Check sheet for the modelled part. Datum: model origin and axes. Units: mm. A direction names the side the tool comes from. Give positions to 0.01 mm unless a question says otherwise; leave off trailing zeros. Order: outer loops, then holes, each group sorted by start corner. A loop starts at its lowest first (then second) coordinate and runs counter-clockwise, first axis right, second up.
```python
from build123d import *

# Parameters (mm, degrees)
F1_DEPTH  = 16
F2_W      = 70
F2_H      = 3
F3_DEPTH  = 2
F4_W      = 50
F4_H      = 14
F5_DEPTH  = 2
F6_R      = 1
F9_DEPTH  = 2
F11_DEPTH = 25
F13_D     = 4
F13_DEPTH = 50
F13_TIP   = 1.2017212381
F14_R     = 3
F14_R_2   = 2
F15_DEPTH = 5
F16_R     = 3


# Not quite as in the source:
# - a pattern or mirror of a feature is missing from the dataset's text; its kind, count and spacing are read off the source's solid


with BuildPart() as f1:
    # F0 (on Front) → F1 (new body)
    with BuildSketch(Plane.XZ):
        with BuildLine():
            Line((94, 11), (0, 11))
            ThreePointArc((0, 11), (-11, 0), (0, -11))
            Line((0, -11), (19, -11))
            ThreePointArc((19, -11), (21.7681124643, -11.8361612201), (23.6103896104, -14.064978646))
            ThreePointArc((23.6103896104, -14.064978646), (47.8977113224, -44.6078392712), (84.5520957277, -57.9942665386))
            ThreePointArc((84.5520957277, -57.9942665386), (89.6419160729, -59.3768457194), (93.8590048523, -62.5444881493))
            Line((93.8590048523, -62.5444881493), (95.1549842887, -61))
            ThreePointArc((95.1549842887, -61), (90.3976747979, -57.5207528796), (84.7034264019, -56))
            ThreePointArc((84.7034264019, -56), (49.0672193413, -42.9854179344), (25.4545454545, -13.2909701044))
            ThreePointArc((25.4545454545, -13.2909701044), (22.87535745, -10.1706257081), (19, -9))
            Line((19, -9), (0, -9))
            ThreePointArc((0, -9), (-9, 0), (0, 9))
            Line((0, 9), (94, 9))
            Line((94, 9), (94, 11))
        make_face()
    extrude(amount=F1_DEPTH)

    # F2 (on face) → F3 (join)
    with BuildSketch(Plane.XY.offset(11)):
        with Locations((59, -17.5)):
            Rectangle(F2_W, F2_H)
    extrude(amount=-F3_DEPTH)

    # F4 (on face) → F5 (join)
    with BuildSketch(Plane.XZ.offset(19)):
        with Locations((69, 4)):
            Rectangle(F4_W, F4_H)
    extrude(amount=-F5_DEPTH)

    # F6
    f6_edges = [f1.edges().sort_by_distance(p)[0] for p in [
        (59, -19, 11),
        (69, -17, 9),
    ]]
    fillet(f6_edges, radius=F6_R)

    # F7: F1 across plane


with BuildPart() as f1_1:
    add(f1.part)
    add(f1.part.mirror(Plane.XZ))

    # F8 (on face) → F9 (cut)
    with BuildSketch(Plane.XY.offset(11)):
        with BuildLine():
            Line((94, 12), (34, 12))
            ThreePointArc((34, 12), (22, 0), (34, -12))
            Line((34, -12), (94, -12))
            Line((94, -12), (94, 12))
        make_face()
    extrude(amount=-F9_DEPTH, mode=Mode.SUBTRACT)

    # F10 (on face) → F11 (cut)
    with BuildSketch(Plane.XZ.offset(19)):
        with BuildLine():
            ThreePointArc((50, 5), (47, 2), (50, -1))
            Line((50, -1), (70, -1))
            ThreePointArc((70, -1), (73, 2), (70, 5))
            Line((70, 5), (50, 5))
        make_face()
    extrude(amount=-F11_DEPTH, mode=Mode.SUBTRACT)

    # F13
    with Locations(Plane.XZ.offset(19)):
        with Locations((80, 3)):
            Hole(F13_D / 2, depth=F13_DEPTH)
            with Locations((0, 0, -(F13_DEPTH + F13_TIP / 2))):  # 118° drill point
                Cone(0, F13_D / 2, F13_TIP, mode=Mode.SUBTRACT)

    # F14 (on face) → F15 (join)
    with BuildSketch(Plane(origin=(0, -17, 0), x_dir=(-1, 0, 0), z_dir=(0, 1, 0))):
        with Locations((-80, 3)):
            Circle(F14_R)
        with Locations((-80, 3)):
            Circle(F14_R_2, mode=Mode.SUBTRACT)
    f15 = extrude(amount=F15_DEPTH)

    # F15_copies: F15 across plane
    add(f15.mirror(Plane.ZX))

    # F16
    f16_edges = [f1_1.edges().sort_by_distance(p)[0] for p in [
        (94, -18, -3),
        (94, 18, -3),
        (44, -18, -3),
        (44, 18, -3),
    ]]
    fillet(f16_edges, radius=F16_R)


solid = f1_1.part
```
(1) Set-up check for faces 1 (the face through (26, 16, -17)), 2 (the face through (9, 0, -11)), 3 (the face through (79, 12, 1)), 4 (the face through (49.505, -0.224, -43.298)), 5 (the face through (26, -16, -17)): record each of +Z, -Z, +X, -X, +Y, -Y from which the full face is reachable in a straight line by a thin tool's end or side.
Response values:
face 1: -Z, -X, +Y
face 2: -Z, -X, +Y, -Y
face 3: +Z, +X
face 4: +X, +Y, -Y
face 5: -Z, -X, -Y
(2) Cross-section at D-D on z = 3. Count the separate pieces of the cut face and the enclosed holes in it, then the cut area to 3 significant figures.
Response values:
separate pieces: 6
enclosed holes: 0
area: 220 mm2
(3) Cross-section at C-C on x = 40.5. Enter the section's corners in (y, z).
Response values:
outline: (-19, 9) - (-12, 9) - (-12, 11) - (-18, 11) arc R1 ccw to (-19, 10) - close; (-16, -38.49) - (16, -38.49) - (16, -35.7) - (-16, -35.7) - close; (12, 9) - (19, 9) - (19, 10) arc R1 ccw to (18, 11) - (12, 11) - close
(4) Release check for a two-part mould opening along Z. For faces 6 (the face through (83, 15, 3)), 7 (the face through (74, -19, 5)), 8 (the face through (-11, 0, 0)) record: released by +Z, released by -Z, zero draft, split by the parting line, or undercut.
Response values:
face 6: undercut
face 7: zero draft
face 8: split by the parting line
(5) Cross-section at B-B on y = 0. Enter the section's corners in (x, z).
Response values:
outline: (0, -11) - (19, -11) arc R5 cw to (23.61, -14.06) arc R72 ccw to (84.55, -57.99) arc R14 cw to (93.86, -62.54) - (95.15, -61) arc R16 ccw to (84.7, -56) arc R70 cw to (25.45, -13.29) arc R7 ccw to (19, -9) - (0, -9) arc R9 cw to (0, 9) - (22, 9) - (22, 11) - (0, 11) arc R11 ccw to start
(6) Gauge pin test, flat ends, axial feed: pin 1 Ø3 at (x, y) = (2, 11) entering from -Z; pin 2 Ø8 at (y, z) = (4.5, -42.5) entering from -X; pin 3 Ø1.6 at (x, y) = (73.5, -18) entering from -Z. Record the tip position at first contact, or that the pin passes through.
Response values:
pin 1: stops at z = -11
pin 2: stops at x = 40.51
pin 3: stops at z = -3
(7) Material ranges on L1, parallel to Z at x = 80, y = -13; L2, parallel to Z at x = 80, y = -17.4; L3, parallel to X at y = 9, z = -24, recorded low to high.
Response values:
L1: z = -57.5 to -55.48, 0 to 1, 5 to 6, 9 to 11
L2: z = -3 to 1, 5 to 11
L3: x = 28.72 to 31.08
(8) Cross-section at A-A on x = 15. Enter the section's corners in (y, z), then the cut area to 3 significant figures.
Response values:
outline: (-16, -11) - (16, -11) - (16, -9) - (-16, -9) - close; (-16, 9) - (16, 9) - (16, 11) - (-16, 11) - close
area: 128 mm2
